Verification items for the finished model (mm, model axes). Face numbers are marked on the shaded views. A direction names the side the tool comes from. Coordinates: 2 decimals unless noted, no trailing zeros. Write each loop counter-clockwise with the first axis right and the second up, starting at its lowest first coordinate (ties: lowest second). Pieces come first, ordered by that corner, then holes. Notation, with made-up numbers: (64.25, 3.25) -> (121.25, 3.25) arc R8 cw to (121.25, 7.25) -> close; hole circle Ø2 at (68.5, 43). An arc over 180 degrees is marked (long way). Answer in a Markdown table with one row per item.
```python
from build123d import *

# Parameters (mm, degrees)
F0_R     = 40.5
F1_DEPTH = 21
F2_R     = 3
F3_DEPTH = 3
F4_R     = 1.5
F5_DEPTH = 25
F7_DEPTH = 9
F8_R     = 3
F9_DEPTH = 20


with BuildPart() as f1:
    # F0 (on Top) → F1 (new body)
    with BuildSketch(Plane.XY):
        Circle(F0_R)
    extrude(amount=F1_DEPTH)

    # F2 (on face) → F3 (cut)
    with BuildSketch(Plane.XY.offset(21)):
        with Locations((-25.5, 0)):
            Circle(F2_R)
        with Locations((25.5, 0)):
            Circle(F2_R)
    extrude(amount=-F3_DEPTH, mode=Mode.SUBTRACT)

    # F4 (on face) → F5 (cut)
    with BuildSketch(Plane.XY.offset(18)):
        with Locations((-25.5, 0)):
            Circle(F4_R)
        with Locations((25.5, 0)):
            Circle(F4_R)
    extrude(amount=-F5_DEPTH, mode=Mode.SUBTRACT)

    # F6 (on face) → F7 (cut)
    with BuildSketch(Plane(origin=(0, 0, 0), x_dir=(1, 0, 0), z_dir=(0, 0, -1))):
        Polygon((2.886751, 5), (-2.886751, 5), (-5.773503, 0), (-2.886751, -5), (2.886751, -5), (5.773503, 0), align=None)
    extrude(amount=-F7_DEPTH, mode=Mode.SUBTRACT)

    # F8 (on face) → F9 (cut)
    with BuildSketch(Plane(origin=(0, 0, 0), x_dir=(1, 0, 0), z_dir=(0, 0, -1))):
        Circle(F8_R)
    extrude(amount=-F9_DEPTH, mode=Mode.SUBTRACT)


solid = f1.part
```
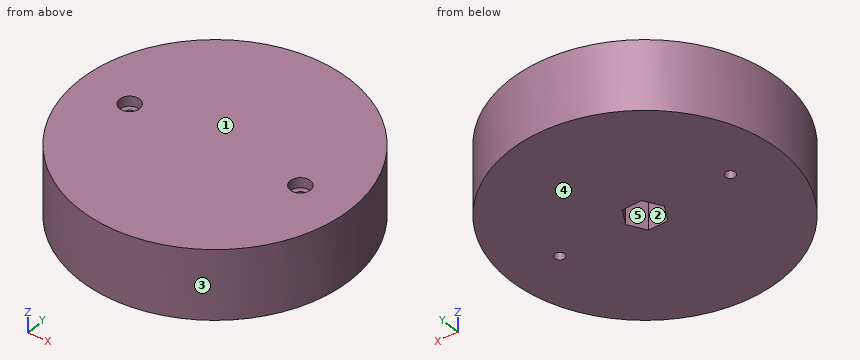
1. Depth check by flat-ended pin: P1, Ø2.5, axis at x = 25.5, y = 0, coming from the -Z side; P2, Ø1.8, axis at x = 0, y = 1, coming from the -Z side; P3, Ø1.5, axis at x = 5.5, y = -24.5, coming from the -Z side; P4, Ø4.5, axis at x = -0.5, z = 5.5, coming from the -Y side. Enter the tip coordinate at first touch or a pass-through.
Geometry says:
| item | result |
|---|---|
| P1 | through |
| P2 | z = 20 |
| P3 | z = 0 |
| P4 | y = -40.5 |
2. Tool access check on the marked faces 4 and 5. Record the directions out of +Z, -Z, +X, -X, +Y, -Y that give a thin tool (end or side, any length) a straight path to the whole face; none if there is none.
Geometry says:
| item | result |
|---|---|
| face 4 | -Z, +X, -X, +Y, -Y |
| face 5 | -Z |
3. Section check D-D, the plane z = 11.75. Record the boundary of the cut face in (x, y), plus the area to 3 significant figures.
Geometry says:
| item | result |
|---|---|
| outline | circle Ø81 at (0, 0); hole circle Ø3 at (-25.5, 0); hole circle Ø6 at (0, 0); hole circle Ø3 at (25.5, 0) |
| area | 5,110 mm^2 |
4. Thickness scan on line 1 (Y direction, x = 0, z = 12.25); line 2 (Y direction, x = 25.5, z = 4.5); line 3 (X direction, y = 12.5, z = 10). Record the ranges inside material, lowest first. Write a range as from..to.
Geometry says:
| item | result |
|---|---|
| line 1 | -40.5..-3, 3..40.5 |
| line 2 | -31.46..-1.5, 1.5..31.46 |
| line 3 | -38.52..38.52 |
5. Mould release check, pull along X, two halves, no side actions. Record for the marked faces 1, 2 and 3: released by +X, released by -X, zero draft, split by the parting line, or undercut.
Geometry says:
| item | result |
|---|---|
| face 1 | zero draft |
| face 2 | undercut |
| face 3 | split by the parting line |
6. Section check C-C, the plane x = 0. Record the boundary of the cut face in (y, z), plus the area to 4 significant figures.
Geometry says:
| item | result |
|---|---|
| outline | (-40.5, 0) -> (-5, 0) -> (-5, 9) -> (-3, 9) -> (-3, 20) -> (3, 20) -> (3, 9) -> (5, 9) -> (5, 0) -> (40.5, 0) -> (40.5, 21) -> (-40.5, 21) -> close |
| area | 1,545 mm^2 |
7. Section check B-B, the plane x = -25.5. Record the boundary of the cut face in (y, z).
Geometry says:
| item | result |
|---|---|
| outline | (-31.46, 0) -> (-1.5, 0) -> (-1.5, 18) -> (-3, 18) -> (-3, 21) -> (-31.46, 21) -> close; (1.5, 0) -> (31.46, 0) -> (31.46, 21) -> (3, 21) -> (3, 18) -> (1.5, 18) -> close |
8. Section check A-A, the plane z = 6.75. Record the boundary of the cut face in (x, y), plus the area to 3 significant figures.
Geometry says:
| item | result |
|---|---|
| outline | circle Ø81 at (0, 0); hole circle Ø3 at (-25.5, 0); hole (-5.77, 0) -> (-2.89, -5) -> (2.89, -5) -> (5.77, 0) -> (2.89, 5) -> (-2.89, 5) -> close; hole circle Ø3 at (25.5, 0) |
| area | 5,050 mm^2 |
